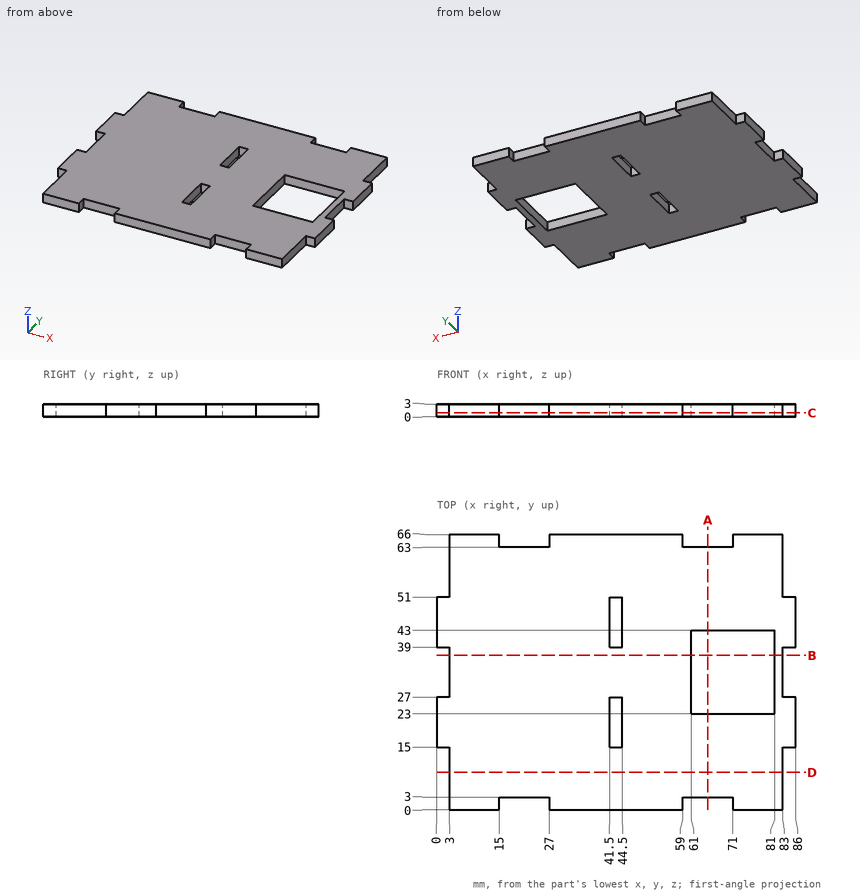
Can you work these out from the drawing? Everything is in mm from the part's minimum corner. Give positions to 0.01 mm unless a question says otherwise; leave off trailing zeros. Loops run counter-clockwise (first coordinate to the right, second up) from the corner with the lowest first, then second, coordinate; pieces in that order, holes last. Notation, with made-up numbers: (33.5, 16) - (53.5, 16) arc R6 ccw to (53.5, 26) - close; hole circle Ø11 at (-8, 66). An arc over 180 degrees is marked (long way). Answer as a JSON object with one key per item and string values.
Q1. Imagine slicing it at B-B on y = 37. Write out the boundary of the cut face in (x, z).
Geometry says:
{"outline": "(3, 0) - (61, 0) - (61, 3) - (3, 3) - close; (81, 0) - (83, 0) - (83, 3) - (81, 3) - close"}
Q2. If I drill on L1, parallel to X at y = 24, z = 2.05; L2, parallel to Y at x = 44, z = 1.95; L3, parallel to X at y = 29.5, z = 0.5, over which ranges is the centre line in solid material (lowest first)?
Geometry says:
{"L1": "0 to 41.5, 44.5 to 61, 81 to 86", "L2": "0 to 15, 27 to 39, 51 to 66", "L3": "3 to 61, 81 to 83"}
Q3. Imagine slicing it at A-A on x = 65. Write out the boundary of the cut face in (y, z), plus the area to 3 significant figures.
Geometry says:
{"outline": "(3, 0) - (23, 0) - (23, 3) - (3, 3) - close; (43, 0) - (63, 0) - (63, 3) - (43, 3) - close", "area": "120 mm²"}
Q4. Will these pins go through, and if not, where does the flat tip stop? P1, Ø1.5, axis at y = 57, z = 1.5, coming from the +X side; P2, Ø1.5, axis at y = 65, z = 1.5, coming from the -X side; P3, Ø1.5, axis at x = 1.5, z = 2, coming from the +Y side.
Geometry says:
{"P1": "x = 83", "P2": "x = 3", "P3": "y = 51"}
Q5. Imagine slicing it at D-D on y = 9. Write out the boundary of the cut face in (x, z), plus the area to 3 significant figures.
Geometry says:
{"outline": "(3, 0) - (83, 0) - (83, 3) - (3, 3) - close", "area": "240 mm²"}
Q6. Imagine slicing it at C-C on z = 0.9. Give the number of separate pieces and of enclosed holes in the cut face, plus the area to 3 significant figures.
Geometry says:
{"separate pieces": "1", "enclosed holes": "3", "area": "4,810 mm²"}
